Design review of the part built by this model. Coordinates are the model's own, in mm. A direction names the side the tool comes from. Give positions to 0.01 mm unless a question says otherwise; leave off trailing zeros. Loops run counter-clockwise (first coordinate to the right, second up) from the corner with the lowest first, then second, coordinate; pieces in that order, holes last. Notation, with made-up numbers: (7.5, 75) - (25.5, 75) arc R34 ccw to (25.5, 112) - close; hole circle Ø6 at (-2, 44). An arc over 180 degrees is marked (long way). Write each question's results on one line, items separated by ' | '.
from build123d import *

# Parameters (mm, degrees)
FILLET1_R = 2


with BuildPart() as part:
    # Sketch1 → Revolve1 (revolve)
    with BuildSketch(Plane(origin=(0, 0, 0), x_dir=(1, 0, 0), z_dir=(0, 1, 0)), mode=Mode.PRIVATE) as revolve1_sk:
        with BuildLine():
            Line((0, 85.203744498), (15, 85.203744498))
            Line((15, 85.203744498), (15, 75.203744498))
            Line((15, 75.203744498), (14, 75.203744498))
            Line((14, 75.203744498), (16.755430859, 56.187296855))
            Line((16.755430859, 56.187296855), (16.805273968, 55.355672424))
            ThreePointArc((16.805273968, 55.355672424), (17.674850572, 47.783264008), (19.362594994, 40.350293442))
            Line((19.362594994, 40.350293442), (20.614214842, 35.960443447))
            ThreePointArc((20.614214842, 35.960443447), (27.100498023, 15.138305045), (34.588001623, -5.345117691))
            Line((34.588001623, -5.345117691), (34.711447428, -5.659018669))
            ThreePointArc((34.711447428, -5.659018669), (36.566659948, -11.769202622), (37.425911626, -18.096749382))
            Line((37.425911626, -18.096749382), (40, -64.796255502))
            Line((40, -64.796255502), (40, -164.796255502))
            ThreePointArc((40, -164.796255502), (37.071067812, -171.867323314), (30, -174.796255502))
            Line((30, -174.796255502), (0, -174.796255502))
            Line((0, -174.796255502), (0, 85.203744498))
        make_face()
    revolve(revolve1_sk.sketch.rotate(Axis((0, 0, -47.713129303), (0, 0, 1)), 180), axis=Axis((0, 0, -47.713129303), (0, 0, 1)))

    # Fillet1
    fillet1_edges = [part.edges().sort_by_distance(p)[0] for p in [
        (15, 0, -85.203744498),
    ]]
    fillet(fillet1_edges, radius=FILLET1_R)


solid = part.part
(1) Tool access review of faces 1 (the flat face through (0, 0, 174.796)), 2 (the cylindrical face through (-8.06, -12.65, -79.15)): name each direction out of +Z, -Z, +X, -X, +Y, -Y from which nothing blocks a thin tool from reaching the whole face with its end or side.
Answers below:
face 1: +Z, +X, -X, +Y, -Y | face 2: -Z
(2) Take a section at A-A on z = 99.5. Give the boundary of the cut face in (x, y).
Answers below:
outline: circle Ø80 at (0, 0)
(3) Draft analysis for pull direction Z (two halves, no side actions). For faces 3 (the flat face through (0, 0, -85.204)), 4 (the cylindrical face through (39.96, -1.76, 115.5)), 5 (the conical face through (11.976, 9.183, -67.675)), state which applies: pulls with the +Z half, pulls with the -Z half, needs draft (parallel to the pull), parting line crosses it, or undercut.
Answers below:
face 3: pulls with the -Z half | face 4: needs draft | face 5: undercut
(4) Wall thickness on line 1 along Y through (x, z) = (0, 132); line 2 along Y through (x, z) = (-13, 62); line 3 along X through (y, z) = (-0.5, 48): over which ranges is each line inside the solid? List them lowest first. Write a range as from..to.
Answers below:
line 1: -40..40 | line 2: -37.67..37.67 | line 3: -39.07..39.07
(5) Insertion check: P1, Ø2, axis at x = 4, z = 42.5, coming from the -Y side; P2, Ø10, axis at y = 15.5, z = 92.5, coming from the -X side; P3, Ø2, axis at y = 11, z = -28, coming from the +X side. Each pin has a flat end and moves straight along its axis. Give the tip position at first contact, or say it passes through.
Answers below:
P1: y = -38.67 | P2: x = -38.6 | P3: x = 20.78
